Build history of the part. All positions in model axes, mm. Face numbers are marked on the shaded views. Give positions to 0.01 mm unless a question says otherwise; leave off trailing zeros. Loops run counter-clockwise (first coordinate to the right, second up) from the corner with the lowest first, then second, coordinate; pieces in that order, holes last. Notation, with made-up numbers: (-31.75, 41) -> (24.25, 41) arc R12 ccw to (24.25, 47) -> close; hole circle Ø7 at (22, 55). An arc over 180 degrees is marked (long way). One line per question, with ' | ' between items. Start each with the question number.
(1) Drill centre lines: L1, parallel to X at y = 115.5, z = -1; L2, parallel to Y at x = 30, z = -10.5; L3, parallel to X at y = 120, z = -5. Where is each one in solid material? Low to high. Write a range as from..to.
(2) Slice it at B-B, the plane x = 30. Write the cut outline in (y, z), then the cut area to 3 significant figures.
(3) Slice it at D-D, the plane y = 116.25. Write the cut outline in (x, z), then the cut area to 3 significant figures.
(4) Slice it at C-C, the plane z = -10.5. Write the cut outline in (x, y), then the cut area to 3 significant figures.
(5) Mould opens along X. For the marked faces 1, 2 and 3 say: pulls with the +X half, pulls with the -X half, needs draft (parallel to the pull), parting line crosses it, or undercut.
(6) Slice it at A-A, the plane y = 120. Write the cut outline in (x, z), then the cut area to 3 significant figures.
(7) Flat gauge pins, fed straight in: pin 1 Ø4 at (y, z) = (118, -8.5) entering from -X; pin 2 Ø2 at (x, y) = (30, 120) entering from +Z (3 decimals); pin 3 Ø2 at (y, z) = (121, -12) entering from +X; pin 4 Ø1.5 at (y, z) = (119.5, -7) entering from -X. Where does each tip first touch, or does it go through?
```python
from build123d import *

# Parameters (mm, degrees)
SKETCH053_R     = 1.25
PAD016_DEPTH    = 14
SKETCH054_W     = 70.5
SKETCH054_H     = 33.8
POCKET031_DEPTH = 1.6
POCKET032_DEPTH = 125.001


with BuildPart() as part:
    # Sketch053 → Pad016 (new body)
    with BuildSketch(Plane.XY):
        with BuildLine():
            ThreePointArc((-40, 125), (-40.353553, 124.853553), (-40.5, 124.5))
            Line((-40.5, 115.5), (-40.5, 124.5))
            ThreePointArc((-40.5, 115.5), (-40.353553, 115.146447), (-40, 115))
            Line((40, 115), (-40, 115))
            ThreePointArc((40, 115), (40.353553, 115.146447), (40.5, 115.5))
            Line((40.5, 124.5), (40.5, 115.5))
            ThreePointArc((40.5, 124.5), (40.353553, 124.853553), (40, 125))
            Line((-40, 125), (40, 125))
        make_face()
        with Locations((-30, 120)):
            Circle(SKETCH053_R, mode=Mode.SUBTRACT)
        with Locations((30, 120)):
            Circle(SKETCH053_R, mode=Mode.SUBTRACT)
    extrude(amount=-PAD016_DEPTH)

    # Sketch054 → Pocket031 (cut)
    with BuildSketch(Plane.XY):
        with Locations((0, 106.9)):
            Rectangle(SKETCH054_W, SKETCH054_H)
    extrude(amount=-POCKET031_DEPTH, mode=Mode.SUBTRACT)

    # Sketch055 → Pocket032 (cut, through all)
    with BuildSketch(Plane.XZ):
        Polygon((-53, 10), (0, -43), (53, 10), (53, -60), (-53, -60), align=None)
    extrude(amount=-POCKET032_DEPTH, mode=Mode.SUBTRACT)


solid = part.part
```
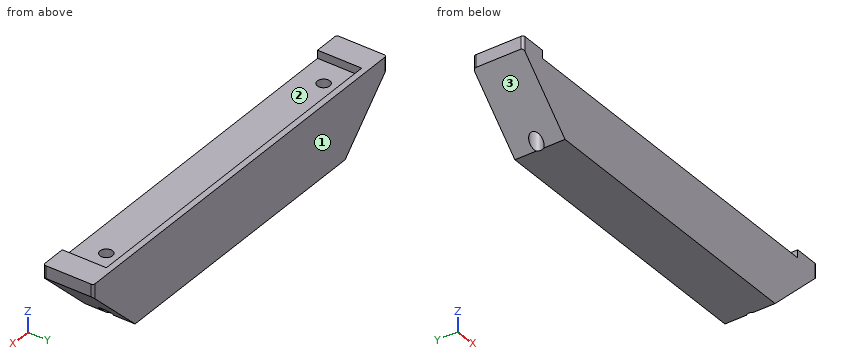
Final values:
1) L1: -40.5..-35.25, 35.25..40.5 | L2: 115..118.75, 121.25..125 | L3: -38..-31.25, -28.75..28.75, 31.25..38
2) outline: (115, -13) -> (118.75, -13) -> (118.75, -1.6) -> (115, -1.6) -> close; (121.25, -13) -> (125, -13) -> (125, 0) -> (123.8, 0) -> (123.8, -1.6) -> (121.25, -1.6) -> close | area: 87.4 mm2
3) outline: (-40.5, -2.5) -> (-29, -14) -> (29, -14) -> (40.5, -2.5) -> (40.5, 0) -> (35.25, 0) -> (35.25, -1.6) -> (-35.25, -1.6) -> (-35.25, 0) -> (-40.5, 0) -> close | area: 889 mm2
4) outline: (-32.5, 115) -> (32.5, 115) -> (32.5, 125) -> (-32.5, 125) -> close; hole circle Ø2.5 at (-30, 120); hole circle Ø2.5 at (30, 120) | area: 640 mm2
5) face 1: needs draft | face 2: undercut | face 3: pulls with the -X half
6) outline: (-40.5, -2.5) -> (-31.25, -11.75) -> (-31.25, -1.6) -> (-35.25, -1.6) -> (-35.25, 0) -> (-40.5, 0) -> close; (-28.75, -14) -> (28.75, -14) -> (28.75, -1.6) -> (-28.75, -1.6) -> close; (31.25, -11.75) -> (40.5, -2.5) -> (40.5, 0) -> (35.25, 0) -> (35.25, -1.6) -> (31.25, -1.6) -> close | area: 832 mm2
7) pin 1: x = -36.5 | pin 2: through | pin 3: x = 32 | pin 4: x = -36.75
